```python
from build123d import *

# Parameters (mm, degrees)
SKETCH1_R           = 1.7
SKETCH1_R_2         = 12.9
BOSS_EXTRUDE1_DEPTH = 3.5
FILLET1_R           = 2.5
FILLET2_R           = 5
BOSS_EXTRUDE2_DEPTH = 7.75
FILLET3_R           = 3
SKETCH3_R           = 3.2
CUT_EXTRUDE1_DEPTH  = 3.1
SKETCH4_R           = 2
CUT_EXTRUDE2_DEPTH  = 1.75
SKETCH5_R           = 0.85
CUT_EXTRUDE3_DEPTH  = 7
CUT_EXTRUDE4_DEPTH  = 2
BOSS_EXTRUDE3_DEPTH = 16
CUT_EXTRUDE5_DEPTH  = 34.12193382


with BuildPart() as part:
    # Sketch1 → Boss-Extrude1 (new body)
    with BuildSketch(Plane.XY):
        Polygon((-19, -8.290371926), (-19, 17.5), (-14.092522712, 26), (14.092522712, 26), (19, 17.5), (19, -8.290371926), (8, -24), (-8, -24), align=None)
        with Locations((-13, 20)):
            Circle(SKETCH1_R, mode=Mode.SUBTRACT)
        with Locations((13, 20)):
            Circle(SKETCH1_R, mode=Mode.SUBTRACT)
        with Locations((0, 1.35)):
            Circle(SKETCH1_R_2, mode=Mode.SUBTRACT)
    extrude(amount=BOSS_EXTRUDE1_DEPTH)

    # Fillet1
    fillet1_edges = [part.edges().sort_by_distance(p)[0] for p in [
        (-12.9, 1.35, 3.5),
    ]]
    fillet(fillet1_edges, radius=FILLET1_R)

    # Fillet2
    fillet2_edges = [part.edges().sort_by_distance(p)[0] for p in [
        (-19, -8.290371926, 1.75),
        (-19, 17.5, 1.75),
        (-14.092522712, 26, 1.75),
        (14.092522712, 26, 1.75),
        (19, 17.5, 1.75),
        (19, -8.290371926, 1.75),
    ]]
    fillet(fillet2_edges, radius=FILLET2_R)

    # Sketch2 → Boss-Extrude2 (add)
    with BuildSketch(Plane.XY.offset(3.5)):
        Polygon((-12.201245229, -18), (-8, -24), (8, -24), (12.201245229, -18), align=None)
    extrude(amount=BOSS_EXTRUDE2_DEPTH)

    # Fillet3
    fillet3_edges = [part.edges().sort_by_distance(p)[0] for p in [
        (0, -18, 3.5),
        (0, -18, 11.25),
    ]]
    fillet(fillet3_edges, radius=FILLET3_R)

    # Sketch3 → Cut-Extrude1 (cut)
    with BuildSketch(Plane.XZ.offset(24)):
        with Locations(Location((-4.25, 7, 0), (0, 0, 270))):
            Circle(SKETCH3_R)
        with Locations(Location((4.25, 7, 0), (0, 0, 270))):
            Circle(SKETCH3_R)
    extrude(amount=-CUT_EXTRUDE1_DEPTH, mode=Mode.SUBTRACT)

    # Sketch4 → Cut-Extrude2 (cut)
    with BuildSketch(Plane.XZ.offset(20.9)):
        with Locations(Location((-4.25, 7, 0), (0, 0, 270))):
            Circle(SKETCH4_R)
        with Locations(Location((4.25, 7, 0), (0, 0, 270))):
            Circle(SKETCH4_R)
    extrude(amount=-CUT_EXTRUDE2_DEPTH, mode=Mode.SUBTRACT)

    # Sketch5 → Cut-Extrude3 (cut)
    with BuildSketch(Plane(origin=(0, 0, 0), x_dir=(-1, 0, 0), z_dir=(0, 0, -1))):
        with Locations((4.25, -20.225)):
            Circle(SKETCH5_R)
        with Locations((-4.25, -20.225)):
            Circle(SKETCH5_R)
    extrude(amount=-CUT_EXTRUDE3_DEPTH, mode=Mode.SUBTRACT)

    # Sketch6 → Cut-Extrude4 (cut)
    with BuildSketch(Plane(origin=(0, 0, 0), x_dir=(-1, 0, 0), z_dir=(0, 0, -1))):
        with BuildLine():
            Line((18.330127019, 18.660254038), (16.598076211, 21.660254038))
            Line((16.598076211, 21.660254038), (15.267949192, 19.356406461))
            ThreePointArc((15.267949192, 19.356406461), (15.068148347, 18.874044551), (15, 18.356406461))
            Line((15, 18.356406461), (15, -6.398579193))
            ThreePointArc((15, -6.398579193), (14.907433901, -6.999990792), (14.638304089, -7.545732065))
            Line((14.638304089, -7.545732065), (7.862801296, -17.222152873))
            ThreePointArc((7.862801296, -17.222152873), (7.147994434, -17.849021666), (6.224497208, -18.075))
            Line((6.224497208, -18.075), (-3.1, -18.075))
            ThreePointArc((-3.1, -18.075), (-4.514213562, -18.660786438), (-5.1, -20.075))
            Line((-5.1, -20.075), (-5.1, -20.225))
            ThreePointArc((-5.1, -20.225), (-4.851040764, -20.826040764), (-4.25, -21.075))
            Line((-4.25, -21.075), (4.25, -21.075))
            Line((4.25, -21.075), (7.786198359, -21.075))
            ThreePointArc((7.786198359, -21.075), (8.709695586, -20.849021666), (9.424502448, -20.222152873))
            Line((9.424502448, -20.222152873), (17.638304089, -8.491628432))
            ThreePointArc((17.638304089, -8.491628432), (17.907433901, -7.945887158), (18, -7.344475559))
            Line((18, -7.344475559), (18, 17.552558883))
            ThreePointArc((18, 17.552558883), (18.068148347, 18.070196973), (18.267949192, 18.552558883))
            Line((18.267949192, 18.552558883), (18.330127019, 18.660254038))
        make_face()
    extrude(amount=-CUT_EXTRUDE4_DEPTH, mode=Mode.SUBTRACT)

    # Sketch7 → Boss-Extrude3 (add)
    with BuildSketch(Plane(origin=(8, 0, 0), x_dir=(0, 0, -1), z_dir=(1, 0, 0))):
        Polygon((-11.25, -24), (-11.25, -24.9), (-10.35, -24), align=None)
        Polygon((-2.75, -24.9), (-3.65, -24), (0, -24), (0, -24.9), align=None)
    extrude(amount=-BOSS_EXTRUDE3_DEPTH)

    # Sketch9 → Cut-Extrude5 (cut, through all)
    with BuildSketch(Plane.XY.offset(3.5)):
        with BuildLine():
            Line((3.2, 23.25), (3.2, 26))
            Line((3.2, 26), (9.4, 26))
            Line((9.4, 26), (9.4, 23.25))
            ThreePointArc((9.4, 23.25), (6.3, 20.15), (3.2, 23.25))
        make_face()
    extrude(amount=-CUT_EXTRUDE5_DEPTH, mode=Mode.SUBTRACT)


solid = part.part
```
Source: CAD feature listing. Evaluate the final solid. Frame: model axes, mm. A direction names the side the tool comes from. Give positions to 0.01 mm unless a question says otherwise; leave off trailing zeros. Order: outer loops, then holes, each group sorted by start corner. A loop starts at its lowest first (then second) coordinate and runs counter-clockwise, first axis right, second up.
(1) Pull-direction query (Z, two-part tool) for faces 6 (the face through (-18, 5, 1)), 7 (the face through (-4, -19.15, 7)), 8 (the face through (-0.2, -17.14, 4.4)), 9 (the face through (13, 7, 0)); classes: +Z half, -Z half, draft (parallel to the pull), parting line (faces both ways), or undercut.
(2) Material intervals for line 1 along X through (y, z) = (-21.75, 7); line 2 along X through (y, z) = (-22, 6.5); line 3 along Y through (x, z) = (2.5, 0.75) (3 decimals), sorted ascending.
(3) Contact query for flat-ended pins moving along their axis: P1, Ø11.5, axis at x = 5, y = -1.5, coming from the +Z side; P2, Ø1.9, axis at x = 4.5, z = 5.5, coming from the -Y side; P3, Ø3, axis at x = 11, y = -4.5, coming from the +Z side; P4, Ø1.9, axis at x = -4, z = 6.5, coming from the -Y side. Output: stop coordinate, or through.
(4) Access query for faces 1 (the face through (-13.5, -14.4, 1)), 2 (the face through (12.304, 5.225, 0.493)), 3 (the face through (4, -19.15, 7)), 4 (the face through (-15.94, 20.52, 0.99)), 5 (the face through (9, 15, 3.5)). Directions: +Z, -Z, +X, -X, +Y, -Y. A direction counts if a zero-diameter tool reaches every point of the face in a straight line with its end or side. Return the directions, or none.
(5) Section query B-B (y = 21). Return the cut outline in (x, z).
(6) Section query C-C (x = 16.5). Return the cut outline in (y, z), plus the area to 3 significant figures.
(7) Section query A-A (y = 1.35). Return the cut outline in (x, z), plus the area to 3 significant figures.
Outcome:
1. face 6: draft
1. face 7: undercut
1. face 8: +Z half
1. face 9: -Z half
2. line 1: x = -9.58 to -7.45, -1.05 to 1.05, 7.45 to 9.58
2. line 2: x = -9.4 to -7.41, -1.09 to 1.09, 7.41 to 9.4
2. line 3: y = -24.9 to -21.075, -18.075 to -11.305, 14.005 to 26
3. P1: passes through
3. P2: stops at y = -20.9
3. P3: stops at z = 3.04
3. P4: stops at y = -19.15
4. face 1: -Z
4. face 2: +Z, -Z
4. face 3: -Y
4. face 4: -Z, -X
4. face 5: +Z, +X, -X, +Y
5. outline: (-16.98, 2) - (-16.22, 2) - (-16.22, 0) - (-14.37, 0) - (-14.37, 3.5) - (-16.98, 3.5) - close; (-11.63, 0) - (4.17, 0) - (4.17, 3.5) - (-11.63, 3.5) - close; (8.43, 0) - (11.63, 0) - (11.63, 3.5) - (8.43, 3.5) - close; (14.37, 0) - (16.98, 0) - (16.98, 3.5) - (14.37, 3.5) - close
6. outline: (-11.86, 0) - (21.83, 0) - (21.83, 3.5) - (-11.86, 3.5) - close
6. area: 118 mm2
7. outline: (-19, 0) - (-18, 0) - (-18, 2) - (-15, 2) - (-15, 0) - (-12.9, 0) - (-12.9, 1) arc R2.5 ccw to (-15.4, 3.5) - (-19, 3.5) - close; (12.9, 0) - (19, 0) - (19, 3.5) - (15.4, 3.5) arc R2.5 ccw to (12.9, 1) - close
7. area: 34.0 mm2
